Work out the finished part from the listing and answer in its coordinate system (mm). Face numbers are marked on the shaded views. A direction names the side the tool comes from. Coordinates: 2 decimals unless noted, no trailing zeros. Order: outer loops, then holes, each group sorted by start corner. A loop starts at its lowest first (then second) coordinate and runs counter-clockwise, first axis right, second up.
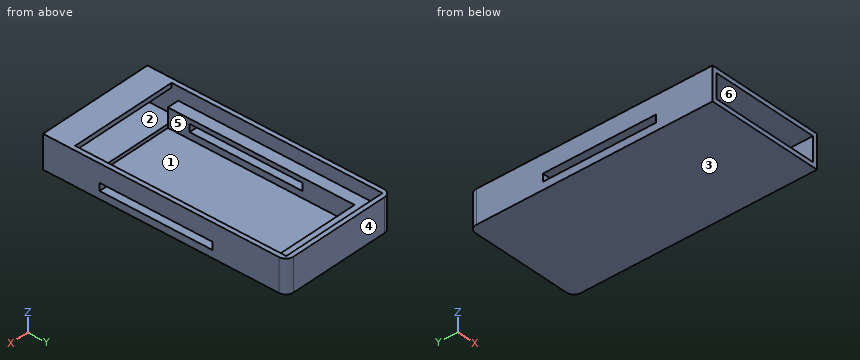
```python
from build123d import *

# Parameters (mm, degrees)
F0_W      = 78.74
F0_H      = 148.336
F1_DEPTH  = 22.225
F2_W      = 72.644
F2_H      = 142.24
F3_DEPTH  = 8.89
F5_DEPTH  = 12.7
F0_H_2    = 15.875
F6_DEPTH  = 22.225
F7_W      = 72.644
F7_H      = 16.129
F8_DEPTH  = 23.447496
F9_W      = 76.2
F9_H      = 5.08
F10_DEPTH = 78.74
F11_R     = 5.08


with BuildPart() as f1:
    # F0 (on Top) → F1 (new body)
    with BuildSketch(Plane.XY):
        with Locations((-6.426373, -1.251059)):
            Rectangle(F0_W, F0_H)
    extrude(amount=F1_DEPTH)

    # F2 (on face) → F3 (cut)
    with BuildSketch(Plane.XY.offset(22.225)):
        with Locations((-6.426373, -1.251059)):
            Rectangle(F2_W, F2_H)
    extrude(amount=-F3_DEPTH, mode=Mode.SUBTRACT)

    # F4 (on face) → F5 (cut)
    with BuildSketch(Plane.XY.offset(13.335)):
        Polygon((-6.426373, 57.940908), (-34.970604, 57.940908), (-34.970604, -67.846563), (22.117858, -67.846563), (22.117858, 57.940908), align=None)
    extrude(amount=-F5_DEPTH, mode=Mode.SUBTRACT)

    # F0 (on Top) → F6 (join)
    with BuildSketch(Plane.XY):
        with Locations((-6.426373, -83.356559)):
            Rectangle(F0_W, F0_H_2)
    extrude(amount=F6_DEPTH)

    # F7 (on face) → F8 (cut, through all)
    with BuildSketch(Plane.XZ.offset(91.294059)):
        with Locations((-6.426373, 11.1125)):
            Rectangle(F7_W, F7_H)
    extrude(amount=-F8_DEPTH, mode=Mode.SUBTRACT)

    # F9 (on face) → F10 (cut, through all)
    with BuildSketch(Plane(origin=(-45.796373, 0, 0), x_dir=(0, -1, 0), z_dir=(-1, 0, 0))):
        with Locations((15.094059, 7.62)):
            Rectangle(F9_W, F9_H)
    extrude(amount=-F10_DEPTH, mode=Mode.SUBTRACT)

    # F11
    f11_edges = [f1.edges().sort_by_distance(p)[0] for p in [
        (-45.796373, 72.916941, 11.1125),
        (32.943627, 72.916941, 11.1125),
    ]]
    fillet(f11_edges, radius=F11_R)


solid = f1.part
```
1. The part is cut by section A-A (x = -16). Determine the outline of the cut face in (y, z) (3 decimals), plus the area to 3 significant figures.
2. The part is cut by section C-C (y = -13). Determine the outline of the cut face in (x, z) (3 decimals), plus the area to 3 significant figures.
3. Consider probe 1 along X at (y, z) = (-64, 8); probe 2 along X at (y, z) = (8.5, 17.25); probe 3 along Z at (x, y) = (-37, -31.5) (3 decimals). Determine where each line is inside the solid, lowest interval first.
4. Flat-ended cylindrical pins translate along their axes: pin 1 (2.5 mm diameter, centred on x = 10.5, z = 16.5, fed in from -Y); pin 2 (12 mm diameter, centred on x = -32, z = 10.5, fed in from -Y). Find the tip coordinate at first contact, or state that the pin passes through.
5. The part is cut by section B-B (z = 8). Determine the outline of the cut face in (x, y), plus the area to 3 significant figures.
6. The mould has two halves that part along Y. Classify the marked faces 4, 5 and 6: released by +Y, released by -Y, zero draft, split by the parting line, or undercut.
7. For the marked faces 1, 2 and 3, determine the directions among +Z, -Z, +X, -X, +Y, -Y from which every point of the face is accessible in a straight line to the end or side of a thin tool.
8. The part is cut by section D-D (y = 42). Determine the outline of the cut face in (x, z) (3 decimals).
Worked out:
1. outline: (-91.294, 0) - (72.917, 0) - (72.917, 22.225) - (69.869, 22.225) - (69.869, 13.335) - (57.941, 13.335) - (57.941, 0.635) - (-67.847, 0.635) - (-67.847, 3.048) - (-91.294, 3.048) - close; (-91.294, 19.177) - (-72.371, 19.177) - (-72.371, 22.225) - (-91.294, 22.225) - close
1. area: 436 mm2
2. outline: (-45.796, 0) - (32.944, 0) - (32.944, 5.08) - (22.118, 5.08) - (22.118, 0.635) - (-34.971, 0.635) - (-34.971, 5.08) - (-45.796, 5.08) - close; (-45.796, 10.16) - (-34.971, 10.16) - (-34.971, 13.335) - (-42.748, 13.335) - (-42.748, 22.225) - (-45.796, 22.225) - close; (22.118, 10.16) - (32.944, 10.16) - (32.944, 22.225) - (29.896, 22.225) - (29.896, 13.335) - (22.118, 13.335) - close
2. area: 269 mm2
3. probe 1: x = -45.8 to -34.97, 22.12 to 32.94
3. probe 2: x = -45.8 to -42.75, 29.9 to 32.94
3. probe 3: z = 0 to 5.08, 10.16 to 13.335
4. pin 1: stops at y = 69.87
4. pin 2: stops at y = -67.85
5. outline: (-45.8, -91.29) - (-42.75, -91.29) - (-42.75, -67.85) - (-34.97, -67.85) - (-34.97, -53.19) - (-45.8, -53.19) - close; (-45.8, 23.01) - (-34.97, 23.01) - (-34.97, 57.94) - (22.12, 57.94) - (22.12, 23.01) - (32.94, 23.01) - (32.94, 67.84) arc R5.08 ccw to (27.86, 72.92) - (-40.72, 72.92) arc R5.08 ccw to (-45.8, 67.84) - close; (22.12, -67.85) - (29.9, -67.85) - (29.9, -91.29) - (32.94, -91.29) - (32.94, -53.19) - (22.12, -53.19) - close
5. area: 2,380 mm2
6. face 4: released by +Y
6. face 5: undercut
6. face 6: zero draft
7. face 1: +Z
7. face 2: -Y
7. face 3: -Z, +X, -X, +Y, -Y
8. outline: (-45.796, 0) - (32.944, 0) - (32.944, 22.225) - (29.896, 22.225) - (29.896, 13.335) - (22.118, 13.335) - (22.118, 0.635) - (-34.971, 0.635) - (-34.971, 13.335) - (-42.748, 13.335) - (-42.748, 22.225) - (-45.796, 22.225) - close
